```python
from build123d import *

# Parameters (mm, degrees)
SKETCH1_W           = 12.7
SKETCH1_H           = 22.86
SKETCH1_R           = 1.65
BOSS_EXTRUDE1_DEPTH = 3.175
SKETCH2_W           = 12.7
SKETCH2_H           = 7.46125
SKETCH2_R           = 1.65
BOSS_EXTRUDE2_DEPTH = 0.889
BOSS_EXTRUDE3_REACH = 19.145
SKETCH3_W           = 0.889
SKETCH3_H           = 0.508
LPATTERN1_COUNT     = 3
LPATTERN1_PITCH     = 2.032
LPATTERN1_COL_COUNT = 3
LPATTERN1_COL_PITCH = 2.032


with BuildPart() as part:
    # Sketch1 → Boss-Extrude1 (new body)
    with BuildSketch(Plane.XY):
        Rectangle(SKETCH1_W, SKETCH1_H)
        with Locations((0, 7.62)):
            Circle(SKETCH1_R, mode=Mode.SUBTRACT)
        with Locations(Location((0, -7.62, 0), (0, 0, 180))):
            Circle(SKETCH1_R, mode=Mode.SUBTRACT)
    extrude(amount=BOSS_EXTRUDE1_DEPTH)

    # Sketch2 → Boss-Extrude2 (add)
    # profile 1 of 2: a face of its own
    with BuildSketch(Plane.XY.offset(3.175)):
        with Locations((0, -7.699375)):
            Rectangle(SKETCH2_W, SKETCH2_H)
        with Locations(Location((0, -7.62, 0), (0, 0, 180))):
            Circle(SKETCH2_R, mode=Mode.SUBTRACT)
    # profile 2 of 2: a face of its own
    with BuildSketch(Plane.XY.offset(3.175)):
        with Locations((0, 7.699375)):
            Rectangle(SKETCH2_W, SKETCH2_H)
        with Locations((0, 7.62)):
            Circle(SKETCH2_R, mode=Mode.SUBTRACT)
    extrude(amount=BOSS_EXTRUDE2_DEPTH)

    # Sketch3 → Boss-Extrude3 (add, up to next)
    with BuildSketch(Plane.XZ.offset(-3.96875), mode=Mode.PRIVATE) as boss_extrude3_sk1:
        with Locations((0, 3.429)):
            Rectangle(SKETCH3_W, SKETCH3_H)
    boss_extrude3_tool1 = extrude(boss_extrude3_sk1.sketch, amount=BOSS_EXTRUDE3_REACH, mode=Mode.PRIVATE) - part.part
    boss_extrude3 = boss_extrude3_tool1.solids().sort_by_distance((0, 3.96875, 3.429))[0]
    add(boss_extrude3)

    # LPattern1: Boss-Extrude3 ×3
    with Locations(*[(i * LPATTERN1_PITCH, 0, 0) for i in range(1, LPATTERN1_COUNT)]):
        add(boss_extrude3)

    # LPattern1 col: Boss-Extrude3 ×3
    with Locations(*[(-i * LPATTERN1_COL_PITCH, 0, 0) for i in range(1, LPATTERN1_COL_COUNT)]):
        add(boss_extrude3)


solid = part.part
```
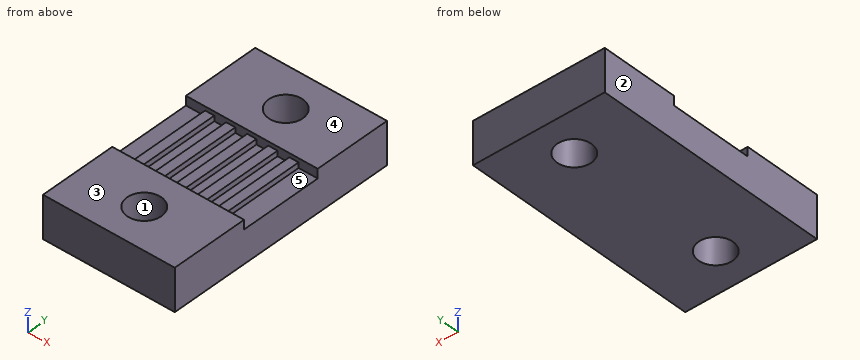
Part model, mm, in its own coordinate system. Face numbers are marked on the shaded views. A direction names the side the tool comes from. Coordinates: 2 decimals unless noted, no trailing zeros. Order: outer loops, then holes, each group sorted by start corner. A loop starts at its lowest first (then second) coordinate and runs counter-clockwise, first axis right, second up. Notation, with made-up numbers: (8, 89.25) - (42, 89.25) arc R20 ccw to (42, 113.25) - close; hole circle Ø1 at (82.25, -22.5). An arc over 180 degrees is marked (long way). Return JSON: item names as keys, results as strings. Group by question number.
Item 1: Which spindle directions (+Z, -Z, +X, -X, +Y, -Y) get a long thin tool onto all of the face, cutting with end or side? Do the marked faces 4 and 5. Say none if no direction does.
Item 2: Pin check, flat tips, straight feed: pin 1 (0.9 mm diameter, centred on x = -3, y = 0.5, fed in from +Z) (3 decimals); pin 2 (0.7 mm diameter, centred on x = -2, y = -0.5, fed in from +Z); pin 3 (2.5 mm diameter, centred on x = 0, y = 7.62, fed in from +Z). Stop position of each tip, or through.
Item 3: Cut at A-A (x = 0). List the corners of the cut face in (y, z).
Item 4: Cut at C-C (y = 7.62). List the corners of the cut face in (x, z), plus the area to 3 significant figures.
Item 5: Drill centre lines: probe 1 along Y at (x, z) = (0, 2.1); probe 2 along X at (y, z) = (-7.62, 2.1); probe 3 along Y at (x, z) = (0.5, 2). Where is each one in solid material? Low to high. Write a range as from..to.
Item 6: Cut at B-B (z = 3.45). State how many separate pieces and enclosed holes the cut face has, plus the area to 3 significant figures.
Item 7: Pull direction X, two halves, no side cores. Call the marked faces 1, 2 and 3: pulls with the +X half, pulls with the -X half, needs draft (parallel to the pull), parting line crosses it, or undercut.
Check values:
{
 "1": {"face 4": "+Z, +X, -X, +Y, -Y", "face 5": "+Z, +X"},
 "2": {"pin 1": "stops at z = 3.175", "pin 2": "stops at z = 3.68", "pin 3": "passes through"},
 "3": {"outline": "(-11.43, 0) - (-9.27, 0) - (-9.27, 4.06) - (-11.43, 4.06) - close; (-5.97, 0) - (5.97, 0) - (5.97, 4.06) - (3.97, 4.06) - (3.97, 3.68) - (-3.97, 3.68) - (-3.97, 4.06) - (-5.97, 4.06) - close; (9.27, 0) - (11.43, 0) - (11.43, 4.06) - (9.27, 4.06) - close"},
 "4": {"outline": "(-6.35, 0) - (-1.65, 0) - (-1.65, 4.06) - (-6.35, 4.06) - close; (1.65, 0) - (6.35, 0) - (6.35, 4.06) - (1.65, 4.06) - close", "area": "38.2 mm2"},
 "5": {"probe 1": "y = -11.43..-9.27, -5.97..5.97, 9.27..11.43", "probe 2": "x = -6.35..-1.65, 1.65..6.35", "probe 3": "y = -11.43..-9.19, -6.05..6.05, 9.19..11.43"},
 "6": {"separate pieces": "1", "enclosed holes": "6", "area": "208 mm2"},
 "7": {"face 1": "undercut", "face 2": "pulls with the -X half", "face 3": "needs draft"}
}
